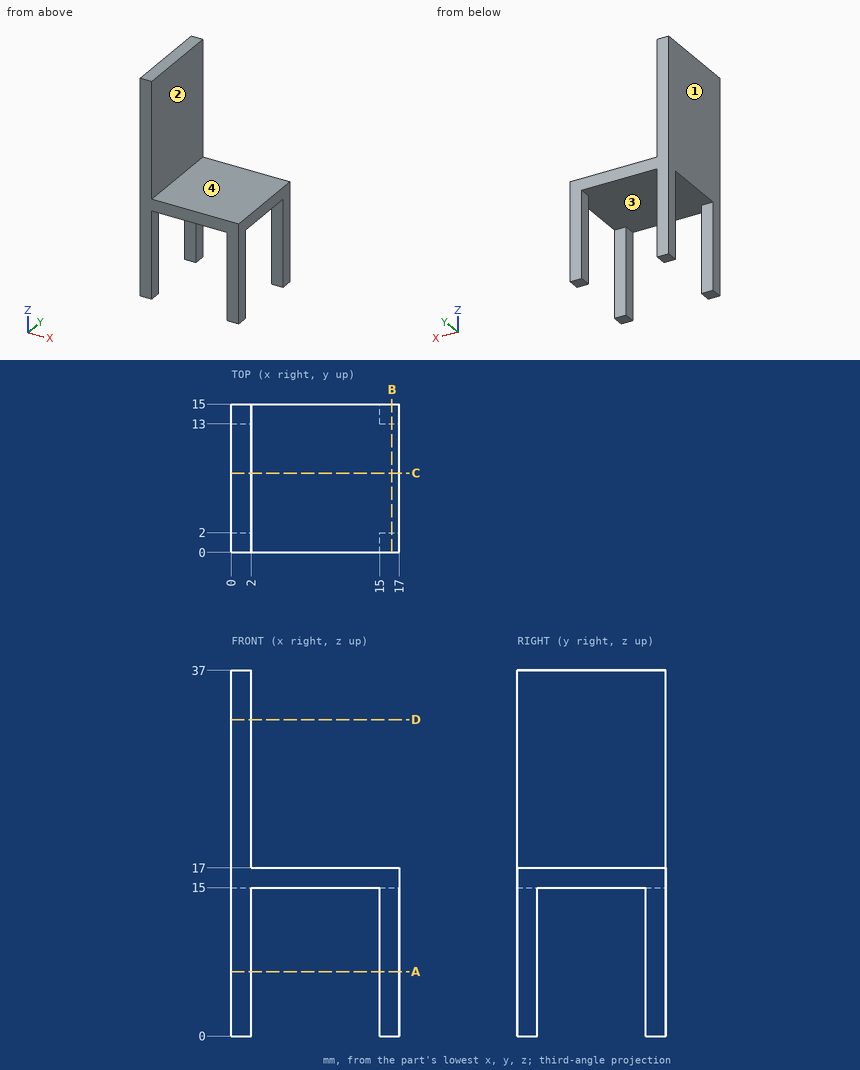
Job drawing, mm, ordinate dimensions from the low corner. One solid piece. Round coordinates to 2 decimals unless told otherwise and drop trailing zeros. Order: outer loops, then holes, each group sorted by start corner. A loop starts at its lowest first (then second) coordinate and runs counter-clockwise, first axis right, second up. Notation, with made-up numbers: (-36.75, 79.25) -> (11.25, 79.25) arc R21 cw to (11.25, 106.25) -> close; hole circle Ø4 at (4, 58.5). An arc over 180 degrees is marked (long way). Answer in a Markdown table with one row per item.
1) Pin check, flat tips, straight feed: P1, Ø0.6, axis at y = 0.5, z = 7.5, coming from the -X side; P2, Ø4.5, axis at y = 8.5, z = 24.5, coming from the +X side; P3, Ø4.5, axis at x = 13, y = 7, coming from the +Z side. Stop position of each tip, or through.
Values:
| item | result |
|---|---|
| P1 | x = 0 |
| P2 | x = 2 |
| P3 | z = 17 |
2) Band-saw the part on C-C on y = 8. Give the cut face in (x, z), and give its area (3 significant figures).
Values:
| item | result |
|---|---|
| outline | (0, 15) -> (17, 15) -> (17, 17) -> (2, 17) -> (2, 37) -> (0, 37) -> close |
| area | 74.0 mm2 |
3) Wall check: L1, parallel to X at y = 0.75, z = 12.5; L2, parallel to Y at x = 16, z = 9; L3, parallel to Z at x = 11, y = 0.75. Give the ranges that are in metal, low to high.
Values:
| item | result |
|---|---|
| L1 | 0 to 2, 15 to 17 |
| L2 | 0 to 2, 13 to 15 |
| L3 | 15 to 17 |
4) Band-saw the part on A-A on z = 6.5. Give the cut face in (x, y), and give its area (3 significant figures).
Values:
| item | result |
|---|---|
| outline | (0, 0) -> (2, 0) -> (2, 2) -> (0, 2) -> close; (0, 13) -> (2, 13) -> (2, 15) -> (0, 15) -> close; (15, 0) -> (17, 0) -> (17, 2) -> (15, 2) -> close; (15, 13) -> (17, 13) -> (17, 15) -> (15, 15) -> close |
| area | 16.0 mm2 |
5) Band-saw the part on B-B on x = 16.25. Give the cut face in (y, z).
Values:
| item | result |
|---|---|
| outline | (0, 0) -> (2, 0) -> (2, 15) -> (13, 15) -> (13, 0) -> (15, 0) -> (15, 17) -> (0, 17) -> close |
6) Band-saw the part on D-D on z = 32. Give the cut face in (x, y).
Values:
| item | result |
|---|---|
| outline | (0, 0) -> (2, 0) -> (2, 15) -> (0, 15) -> close |
7) Mould opens along X. For the marked faces 1, 2, 3 and 4 say: released by +X, released by -X, zero draft, split by the parting line, or undercut.
Values:
| item | result |
|---|---|
| face 1 | released by -X |
| face 2 | released by +X |
| face 3 | undercut |
| face 4 | zero draft |
